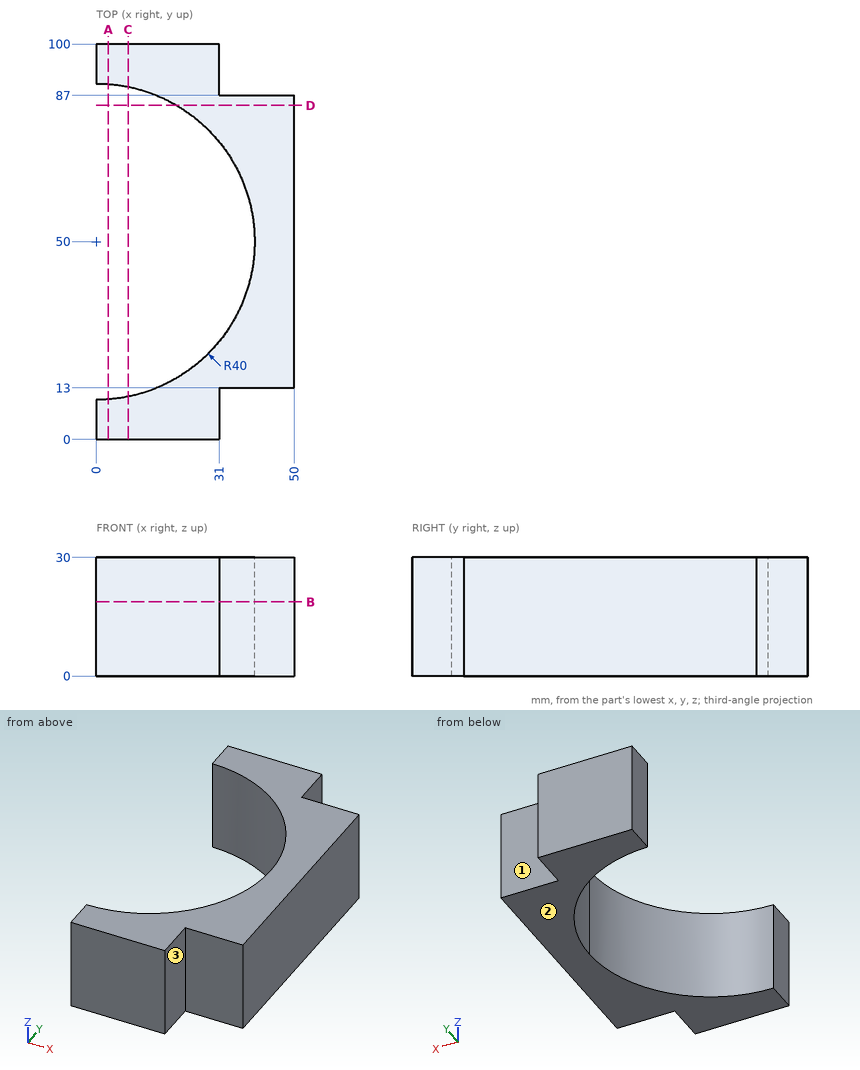
Answer from the drawing. Dimensions are ordinates in mm from the lowest x, y and z of the part. A direction names the side the tool comes from. Coordinates: 2 decimals unless noted, no trailing zeros. Loops run counter-clockwise (first coordinate to the right, second up) from the corner with the lowest first, then second, coordinate; pieces in that order, holes last. Notation, with made-up numbers: (44.5, 55) -> (80.5, 55) arc R29 ccw to (80.5, 85) -> close; hole circle Ø4 at (31.25, 83). An arc over 180 degrees is marked (long way). Answer in a Markdown table with one row per item.
Item 1: Straight lines are drawn through the part: line 1 along Y through (x, z) = (44, 25.75); line 2 along Y through (x, z) = (34.5, 15); line 3 along Y through (x, z) = (6, 5.75). For each, find the intervals that lie inside material, in ascending order. Write a range as [from, to].
Returned:
| item | result |
|---|---|
| line 1 | y = [13, 87] |
| line 2 | y = [13, 29.76], [70.24, 87] |
| line 3 | y = [0, 10.45], [89.55, 100] |
Item 2: A cutting plane is placed at D-D on y = 84.5. Determine the outline of the cut face in (x, z).
Returned:
| item | result |
|---|---|
| outline | (20.24, 0) -> (50, 0) -> (50, 30) -> (20.24, 30) -> close |
Item 3: Each of these flat-tipped pins is pushed along its axis until it touches: P1, Ø2, axis at y = 84, z = 24, coming from the -X side; P2, Ø1.5, axis at y = 34.5, z = 25.5, coming from the -X side; P3, Ø12, axis at x = 10.5, z = 18, coming from the -Y side; P4, Ø4, axis at y = 9, z = 20.5, coming from the +X side. Where does it stop, or does it pass through?
Returned:
| item | result |
|---|---|
| P1 | stops at x = 19.36 |
| P2 | stops at x = 36.55 |
| P3 | stops at y = 0 |
| P4 | stops at x = 31 |
Item 4: A cutting plane is placed at B-B on z = 18.75. Determine the outline of the cut face in (x, y).
Returned:
| item | result |
|---|---|
| outline | (0, 0) -> (31, 0) -> (31, 13) -> (50, 13) -> (50, 87) -> (31, 87) -> (31, 100) -> (0, 100) -> (0, 90) arc R40 cw to (0, 10) -> close |
Item 5: A cutting plane is placed at C-C on x = 8. Determine the outline of the cut face in (y, z).
Returned:
| item | result |
|---|---|
| outline | (0, 0) -> (10.81, 0) -> (10.81, 30) -> (0, 30) -> close; (89.19, 0) -> (100, 0) -> (100, 30) -> (89.19, 30) -> close |
Item 6: A cutting plane is placed at A-A on x = 3. Determine the outline of the cut face in (y, z).
Returned:
| item | result |
|---|---|
| outline | (0, 0) -> (10.11, 0) -> (10.11, 30) -> (0, 30) -> close; (89.89, 0) -> (100, 0) -> (100, 30) -> (89.89, 30) -> close |
Item 7: For the marked faces 1, 2 and 3, determine the directions among +Z, -Z, +X, -X, +Y, -Y from which every point of the face is accessible in a straight line to the end or side of a thin tool.
Returned:
| item | result |
|---|---|
| face 1 | +Z, -Z, +X, +Y |
| face 2 | -Z, +X, -X, +Y, -Y |
| face 3 | +Z, -Z, +X, -Y |
